Verification items for the finished model (mm, model axes). A direction names the side the tool comes from. Round coordinates to 2 decimals unless told otherwise and drop trailing zeros. Loops run counter-clockwise (first coordinate to the right, second up) from the corner with the lowest first, then second, coordinate; pieces in that order, holes last. Notation, with made-up numbers: (-31.5, 1.5) -> (16.5, 1.5) arc R15 cw to (16.5, 6.5) -> close; hole circle Ø11 at (-20, 71.5). An arc over 180 degrees is marked (long way). Use a Markdown table: item, result. Add a question column.
```python
from build123d import *

# Parameters (mm, degrees)
EXTRUDE_1_DEPTH     = 4.5
FILLET_1_R          = 20
SKETCH_2_W          = 10
SKETCH_2_H          = 10
CUT_EXTRUDE_1_DEPTH = 116.19657113


with BuildPart() as part:
    # 스케치1 → 보스-돌출1 (new body)
    with BuildSketch(Plane(origin=(0, 0, 0), x_dir=(1, 0, 0), z_dir=(0, 1, 0))):
        with BuildLine():
            Line((-65, 25), (-34.194351712, 75.754428709))
            ThreePointArc((-34.194351712, 75.754428709), (0, 95), (34.194351712, 75.754428709))
            Line((34.194351712, 75.754428709), (65, 25))
            Line((65, 25), (65, -75))
            Line((65, -75), (-65, -75))
            Line((-65, -75), (-65, 25))
        make_face()
    extrude(amount=EXTRUDE_1_DEPTH)

    # 필렛1
    fillet_1_edges = [part.edges().sort_by_distance(p)[0] for p in [
        (-65, 2.25, -25),
        (65, 2.25, -25),
    ]]
    fillet(fillet_1_edges, radius=FILLET_1_R)

    # 스케치2 → 컷-돌출1 (cut, through all)
    with BuildSketch(Plane(origin=(0, 4.5, 0), x_dir=(1, 0, 0), z_dir=(0, 1, 0))):
        with Locations((-60, 10)):
            Rectangle(SKETCH_2_W, SKETCH_2_H)
        with Locations((60, 10)):
            Rectangle(SKETCH_2_W, SKETCH_2_H)
    extrude(amount=-CUT_EXTRUDE_1_DEPTH, mode=Mode.SUBTRACT)


solid = part.part
```
1) Thickness scan on line 1 (Z direction, x = -42.5, y = 4.2); line 2 (Z direction, x = 15.5, y = 0.65); line 3 (X direction, y = 2.9, z = -64). Record the ranges inside material, lowest first.
2) Sectioned sample at A-A on y = 1.3. Enter the section's corners in (x, z).
3) Sectioned sample at C-C on z = -11. Enter the section's corners in (x, y).
4) Sectioned sample at B-B on x = -32. Enter the section's corners in (y, z), then the cut area to 3 significant figures.
5) Release check for a two-part mould opening along Z. For faces 1 (the face through (60, 2, -5)), 2 (the face through (-0.574, 2.218, -94.996)), 3 (the face through (-65, 2, -17)) record: released by +Z, released by -Z, zero draft, split by the parting line, or undercut.
6) Go/stop test with flat-tipped pins: pin 1 (1.3 mm diameter, centred on y = 1.5, z = -9, fed in from -X); pin 2 (1.5 mm diameter, centred on x = -44.5, z = 11, fed in from -Y); pin 3 (2 mm diameter, centred on x = 61.5, y = 3.5, fed in from -Z); pin 4 (1.3 mm diameter, centred on x = -61.5, y = 1.5, fed in from -Z). Record where each tip stops, or that it passes through.
7) Access from +Z, -Z, +X, -X, +Y, -Y to the whole of each face (thin tool, end or side, straight path). Record for faces 4 (the face through (60, 2, -15)), 5 (the face through (-65, 2, 36)), 6 (the face through (-60, 2, -5)).
Geometry results:
| question | item | result |
|---|---|---|
| 1 | line 1 | -62.07 to 75 |
| 1 | line 2 | -91.87 to 75 |
| 1 | line 3 | -41.33 to 41.33 |
| 2 | outline | (-65, -19.41) arc R20 ccw to (-62.1, -29.78) -> (-34.19, -75.75) arc R40 ccw to (34.19, -75.75) -> (62.1, -29.78) arc R20 ccw to (65, -19.41) -> (65, -15) -> (55, -15) -> (55, -5) -> (65, -5) -> (65, 75) -> (-65, 75) -> (-65, -5) -> (-55, -5) -> (-55, -15) -> (-65, -15) -> close |
| 3 | outline | (-55, 0) -> (55, 0) -> (55, 4.5) -> (-55, 4.5) -> close |
| 4 | outline | (0, -79) -> (4.5, -79) -> (4.5, 75) -> (0, 75) -> close |
| 4 | area | 693 mm^2 |
| 5 | face 1 | undercut |
| 5 | face 2 | released by -Z |
| 5 | face 3 | zero draft |
| 6 | pin 1 | x = -55 |
| 6 | pin 2 | y = 0 |
| 6 | pin 3 | z = -32.41 |
| 6 | pin 4 | z = -31.84 |
| 7 | face 4 | +X, +Y, -Y |
| 7 | face 5 | +Z, -Z, -X, +Y, -Y |
| 7 | face 6 | -X, +Y, -Y |
